from build123d import *

# Parameters (mm, degrees)
EXTRUDE_1_DEPTH = 85
EXTRUDE_START   = -5
EXTRUDE_2_DEPTH = 5
SKETCH_3_W      = 3.820447187
SKETCH_3_H      = 5
EXTRUDE_3_DEPTH = 5
EXTRUDE_4_DEPTH = 5
SKETCH_5_W      = 3.820447187
SKETCH_5_H      = 5
EXTRUDE_5_DEPTH = 5


with BuildPart() as part:
    # Эскиз1 → Бобышка-Вытянуть1 (new body)
    with BuildSketch(Plane(origin=(0, 0, 0), x_dir=(-1, 0, 0), z_dir=(0, 0, -1))):
        with BuildLine():
            Line((-36.94590636, 15.329709821), (-39.102429551, 15.329709821))
            ThreePointArc((-39.102429551, 15.329709821), (-42, 0), (-39.102429551, -15.329709821))
            Line((-39.102429551, -15.329709821), (-36.94590636, -15.329709821))
            ThreePointArc((-36.94590636, -15.329709821), (-40, 0), (-36.94590636, 15.329709821))
        make_face()
    extrude(amount=-EXTRUDE_1_DEPTH)

    # Эскиз2 → Бобышка-Вытянуть2 (add)
    with BuildSketch(Plane.XY.offset(85).offset(EXTRUDE_START)):
        with BuildLine():
            Line((36.94590636, 15.329709821), (36.94590636, 14.329709821))
            Line((36.94590636, 14.329709821), (32.102429551, 14.329709821))
            Line((32.102429551, 14.329709821), (32.102429551, 9.329709821))
            Line((32.102429551, 9.329709821), (38.896741697, 9.329709821))
            ThreePointArc((38.896741697, 9.329709821), (38.039805679, 12.368232853), (36.94590636, 15.329709821))
        make_face()
    extrude(amount=EXTRUDE_2_DEPTH)

    # Эскиз3 → Бобышка-Вытянуть3 (add)
    with BuildSketch(Plane.XY.offset(85)):
        with Locations((34.012653144, 11.829709821)):
            Rectangle(SKETCH_3_W, SKETCH_3_H)
    extrude(amount=EXTRUDE_3_DEPTH)

    # Эскиз4 → Бобышка-Вытянуть4 (add)
    with BuildSketch(Plane.XY.offset(85).offset(EXTRUDE_START)):
        with BuildLine():
            Line((32.102429551, -14.329709821), (36.94590636, -14.329709821))
            Line((36.94590636, -14.329709821), (36.94590636, -15.329709821))
            ThreePointArc((36.94590636, -15.329709821), (38.039805679, -12.368232853), (38.896741697, -9.329709821))
            Line((38.896741697, -9.329709821), (32.102429551, -9.329709821))
            Line((32.102429551, -9.329709821), (32.102429551, -14.329709821))
        make_face()
    extrude(amount=EXTRUDE_4_DEPTH)

    # Эскиз5 → Бобышка-Вытянуть5 (add)
    with BuildSketch(Plane.XY.offset(85)):
        with Locations((34.012653144, -11.829709821)):
            Rectangle(SKETCH_5_W, SKETCH_5_H)
    extrude(amount=EXTRUDE_5_DEPTH)


solid = part.part
Source: CAD feature listing. Evaluate the final solid. Frame: model axes, mm. A direction names the side the tool comes from. Round coordinates to 2 decimals unless told otherwise and drop trailing zeros. Write each loop counter-clockwise with the first axis right and the second up, starting at its lowest first coordinate (ties: lowest second). Pieces come first, ordered by that corner, then holes. Notation, with made-up numbers: (6, -20.5) - (51, -20.5) arc R8 cw to (51, -7.5) - close; hole circle Ø2 at (-28, 12.25). An arc over 180 degrees is marked (long way). Use CSV: the item, a comma, the result in double quotes. Start each with the question number.
(1) Cut plane B-B, the plane y = 0. Return loops of the section in (x, z), and give its area (3 significant figures).
(2) Mould query, pull axis Y, two halves, no side actions, for faces 4 (the face through (32.102, 12, 85)), 5 (the face through (35, 9.33, 84)), 6 (the face through (34, 14.33, 85)), 7 (the face through (38, -15.33, 42)). Classes: pulls with the +Y half, pulls with the -Y half, needs draft (parallel to the pull), parting line crosses it, or undercut.
(3) Set-up query: faces 1 (the face through (35, -9.33, 84)), 2 (the face through (35, -12, 80)), 3 (the face through (35.923, -12, 87)). Return all of +Z, -Z, +X, -X, +Y, -Y with unobstructed straight access to the full face (end or side cutting, diameter ignored); none if empty.
(4) Cut plane D-D, the plane y = 13. Return loops of the section in (x, z).
(5) Cut plane A-A, the plane x = 33. Return loops of the section in (y, z).
(6) Cut plane C-C, the plane z = 34. Return loops of the section in (x, y).
(7) Material intervals for probe 1 along Y at (x, z) = (37, 81); probe 2 along Z at (x, y) = (39.25, 11); probe 3 along Z at (x, y) = (38, -12), sorted ascending. Write a range as [from, to].
(8) First-contact query: pin 1 Ø1.8 at (x, y) = (37, -13) entering from -Z; pin 2 Ø1.5 at (x, z) = (35, 85) entering from +Y; pin 3 Ø1.5 at (y, z) = (12.5, 87.5) entering from +X; pin 4 Ø10 at (y, z) = (8.5, 10.5) entering from -X. Flat tips, straight axial feed; report the tip coordinate or a pass-through.
Geometry says:
1,outline,"(40, 0) - (42, 0) - (42, 85) - (40, 85) - close"
1,area,"170 mm²"
2,face 4,"needs draft"
2,face 5,"undercut"
2,face 6,"pulls with the +Y half"
2,face 7,"pulls with the -Y half"
3,face 1,"+Z, -Z, -X"
3,face 2,"-Z, -X"
3,face 3,"+Z, +X, +Y, -Y"
4,outline,"(32.1, 80) - (37.83, 80) - (37.83, 0) - (39.94, 0) - (39.94, 85) - (35.92, 85) - (35.92, 90) - (32.1, 90) - close"
5,outline,"(-14.33, 80) - (-9.33, 80) - (-9.33, 90) - (-14.33, 90) - close; (9.33, 80) - (14.33, 80) - (14.33, 90) - (9.33, 90) - close"
6,outline,"(36.95, -15.33) - (39.1, -15.33) arc R42 ccw to (39.1, 15.33) - (36.95, 15.33) arc R40 cw to start"
7,probe 1,"[-15.33, -9.33], [9.33, 15.33]"
7,probe 2,"[0, 85]"
7,probe 3,"[80, 85]"
8,pin 1,"z = 0"
8,pin 2,"y = 14.33"
8,pin 3,"x = 35.92"
8,pin 4,"x = 37.65"
